Here's the drawing with two shaded views (mm, measured from the low corner). I have some questions. A direction names the side the tool comes from. Round coordinates to 2 decimals unless told otherwise and drop trailing zeros. Order: outer loops, then holes, each group sorted by start corner. A loop starts at its lowest first (then second) coordinate and runs counter-clockwise, first axis right, second up. Notation, with made-up numbers: (-1.5, -34) - (46.5, -34) arc R30 ccw to (46.5, -5) - close; hole circle Ø11 at (-15.75, 61.5). An arc over 180 degrees is marked (long way). One line per item, written item: value.
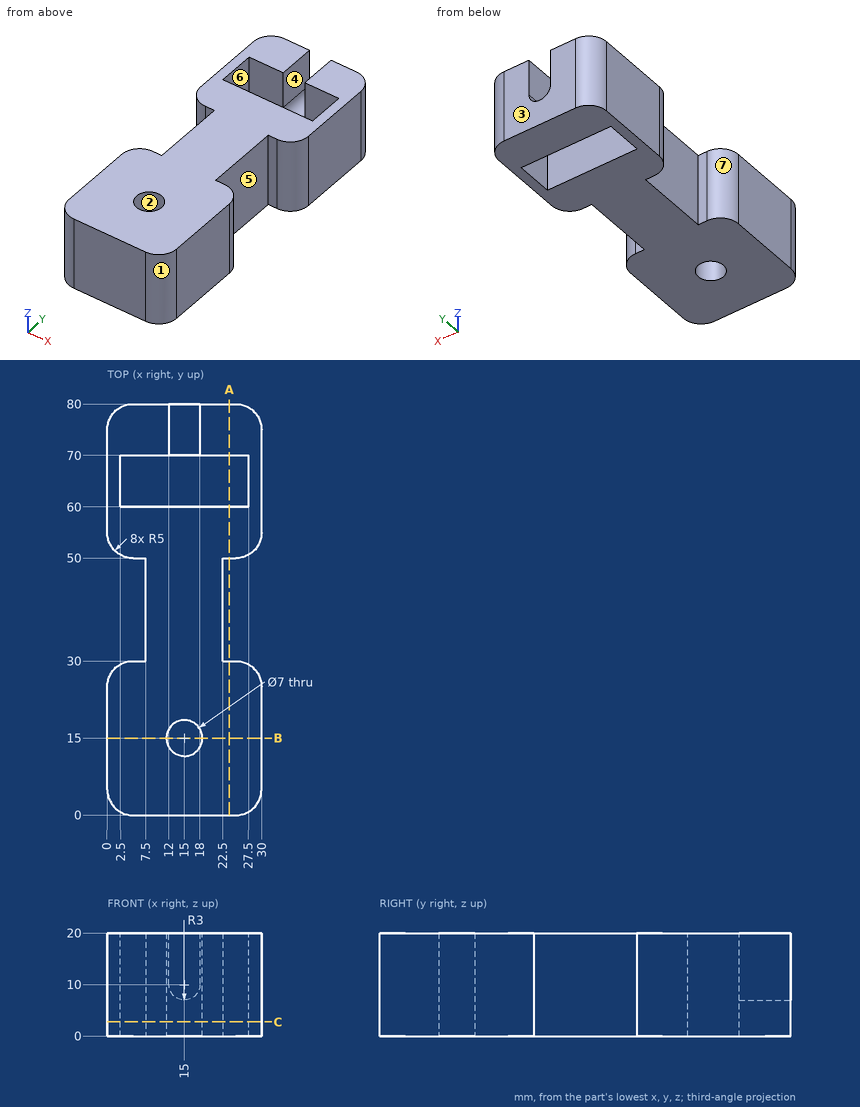
Q1. If I drill on line 1 along Y through (x, z) = (6.25, 9); line 2 along Y through (x, z) = (15, 5); line 3 along Y through (x, z) = (20.5, 10.25), over which ranges is the centre line in solid material (lowest first)?
Results list:
line 1: 0 to 30, 50 to 60, 70 to 80
line 2: 0 to 11.5, 18.5 to 60, 70 to 80
line 3: 0 to 60, 70 to 80
Q2. If we section it at C-C, the plane z = 2.75: Please give me the cut outline in (x, y).
Results list:
outline: (0, 5) arc R5 ccw to (5, 0) - (25, 0) arc R5 ccw to (30, 5) - (30, 25) arc R5 ccw to (25, 30) - (22.5, 30) - (22.5, 50) - (25, 50) arc R5 ccw to (30, 55) - (30, 75) arc R5 ccw to (25, 80) - (5, 80) arc R5 ccw to (0, 75) - (0, 55) arc R5 ccw to (5, 50) - (7.5, 50) - (7.5, 30) - (5, 30) arc R5 ccw to (0, 25) - close; hole (2.5, 60) - (27.5, 60) - (27.5, 70) - (2.5, 70) - close; hole circle Ø7 at (15, 15)
Q3. Will this pin go through, and if not, where does the flat tip stop? pin 1 (3 mm diameter, centred on x = 16, z = 18, fed in from +Y).
Results list:
pin 1: y = 60
Q4. If we section it at A-A, the plane x = 23.75: Please give me the cut outline in (y, z), then the cut area to 3 significant figures.
Results list:
outline: (0, 0) - (30, 0) - (30, 20) - (0, 20) - close; (50, 0) - (60, 0) - (60, 20) - (50, 20) - close; (70, 0) - (80, 0) - (80, 20) - (70, 20) - close
area: 1,000 mm²
Q5. Which directions (+Z, -Z, +X, -X, +Y, -Y) give clear straight access to the entire face, cutting with the end or side of a thin tool? Please do the marked faces 4, 5, 6 and 7.
Results list:
face 4: +Z, +Y
face 5: +Z, -Z, +X
face 6: +Z, -Z
face 7: +Z, -Z, -X
Q6. We'd pull the mould along X, two halves only. Please class the marked faces 1, 2 and 3: released by +X, released by -X, zero draft, split by the parting line, or undercut.
Results list:
face 1: released by +X
face 2: undercut
face 3: zero draft
Q7. If we section it at B-B, the plane y = 15: Please give me the cut outline in (x, z), then the cut area to 3 significant figures.
Results list:
outline: (0, 0) - (11.5, 0) - (11.5, 20) - (0, 20) - close; (18.5, 0) - (30, 0) - (30, 20) - (18.5, 20) - close
area: 460 mm²
